Build history of the part. All positions in model axes, mm. A direction names the side the tool comes from. Give positions to 0.01 mm unless a question says otherwise; leave off trailing zeros. Order: outer loops, then holes, each group sorted by start corner. A loop starts at its lowest first (then second) coordinate and runs counter-clockwise, first axis right, second up. Notation, with made-up numbers: (86, 21.5) - (93, 21.5) arc R8 ccw to (93, 32.5) - close; hole circle Ø11 at (72, 79). An arc over 180 degrees is marked (long way). Write each question's results on one line, items separated by ' | '. Start each with the question number.
1) Drill centre lines: line 1 along Z through (x, y) = (-18, 3.5); line 2 along X through (y, z) = (3, 65.5); line 3 along Z through (x, y) = (-27.5, -19). Where is each one in solid material? Low to high. Write a range as from..to.
2) Cut at A-A on x = -10. List the corners of the cut face in (y, z) (3 decimals).
3) Tool access for faces 4 (the face through (40, -17, -33.732)), 5 (the face through (40, 19, -33.732)), 6 (the face through (-16, -22.225, 86)): list every direction of +Z, -Z, +X, -X, +Y, -Y with a clear straight run to the whole face (end or side of a thin tool).
4) Cut at B-B on y = -19. List the corners of the cut face in (x, z), plus the area to 3 significant figures.
5) Two-plate mould, pull along Y, no slides. Class faces 1 (the face through (65.825, 0, -37)), 2 (the face through (42.605, -12.686, -37.77)), 3 (the face through (30, 4.445, 5)): +Y half, -Y half, draft (parallel to the pull), parting line (faces both ways), or undercut.
6) Drop flat-ended pins along their axis: pin 1 Ø2 at (x, y) = (50, 18.5) entering from +Z; pin 2 Ø21.5 at (x, z) = (25, 38.5) entering from +Y (3 decimals); pin 3 Ø3 at (x, y) = (40.91, 14.92) entering from -Z; pin 4 Ø1.9 at (y, z) = (-6, -36.5) entering from -X. Give the stop position or say it passes through.
7) Cut at C-C on x = -25. List the corners of the cut face in (y, z) (3 decimals).
from build123d import *

# Parameters (mm, degrees)
F0_W           = 50.8
F0_H           = 6.35
F1_DEPTH       = 25.4
F2_DEPTH       = 4.445
F3_R           = 19.05
F4_DEPTH       = 22.225
F5_R           = 15.7047598919
F6_DEPTH       = 44.45
F8_D           = 3.4
F8_CSINK_D     = 6.72
F8_CSINK_ANGLE = 90
F9_D           = 3.4
F9_CSINK_D     = 6.72
F9_CSINK_ANGLE = 90


with BuildPart() as f1:
    # F0 (on Front) → F1 (new body, symmetric)
    with BuildSketch(Plane.XZ):
        with Locations((40.4247476995, -36.9068052319)):
            Rectangle(F0_W, F0_H)
    extrude(amount=F1_DEPTH, both=True)

    # F0 (on Front) → F2 (join, symmetric)
    with BuildSketch(Plane.XZ):
        with Locations((40.4247476995, -36.9068052319)):
            Rectangle(F0_W, F0_H)
        with BuildLine():
            Line((15.0247476995, -33.7318052319), (65.8247476995, -33.7318052319))
            add(Edge.make_bspline(
                [(15.0247476995, -33.7318052319), (12.2795119362, -9.1876940642), (29.4644343196, 7.3717802798), (-44.7611190361, 108.9306998857), (54.9041464645, 15.0382978493), (65.8247476995, -33.7318052319)],
                knots=[0, 0, 0, 0, 0.2744626476, 0.5653253519, 1, 1, 1, 1], degree=3))
        make_face()
    extrude(amount=F2_DEPTH, both=True)

    # F3 (on Front) → F4 (join, symmetric)
    with BuildSketch(Plane.XZ):
        with Locations((-18.4505134821, 70.2780410647)):
            Circle(F3_R)
    extrude(amount=F4_DEPTH, both=True)

    # F5 (on face) → F6 (cut)
    with BuildSketch(Plane.XZ.offset(22.225)):
        with Locations((-18.4505134821, 70.2780410647)):
            Circle(F5_R)
    extrude(amount=-F6_DEPTH, mode=Mode.SUBTRACT)

    # F8 (through all)
    with Locations(Plane.XY.offset(-33.7318052319)):
        with Locations((40.906753391, 14.9225)):
            CounterSinkHole(F8_D / 2, F8_CSINK_D / 2, counter_sink_angle=F8_CSINK_ANGLE)

    # F9 (through all)
    with Locations(Plane.XY.offset(-33.7318052319)):
        with Locations((40.906753391, -12.7611579373)):
            CounterSinkHole(F9_D / 2, F9_CSINK_D / 2, counter_sink_angle=F9_CSINK_ANGLE)


solid = f1.part
Results:
1) line 1: 51.23..54.58, 85.98..89.32 | line 2: -36.89..-33.41, -3.49..-0.01 | line 3: 53.51..57.44, 83.11..87.04
2) outline: (-22.225, 53.205) - (22.225, 53.205) - (22.225, 57.041) - (-22.225, 57.041) - close; (-22.225, 83.515) - (22.225, 83.515) - (22.225, 87.351) - (-22.225, 87.351) - close
3) face 4: +Z, +X, -X, -Y | face 5: +Z, +X, -X, +Y | face 6: +Z, -Z, +X, -X, -Y
4) outline: circle Ø38.1 at (-18.45, 70.28); (15.02, -40.08) - (65.82, -40.08) - (65.82, -33.73) - (15.02, -33.73) - close; hole circle Ø31.41 at (-18.45, 70.28) | area: 688 mm^2
5) face 1: draft | face 2: undercut | face 3: +Y half
6) pin 1: z = -33.73 | pin 2: y = 4.445 | pin 3: through | pin 4: x = 15.02
7) outline: (-22.225, 52.389) - (22.225, 52.389) - (22.225, 56.004) - (-22.225, 56.004) - close; (-22.225, 84.552) - (22.225, 84.552) - (22.225, 88.167) - (-22.225, 88.167) - close
